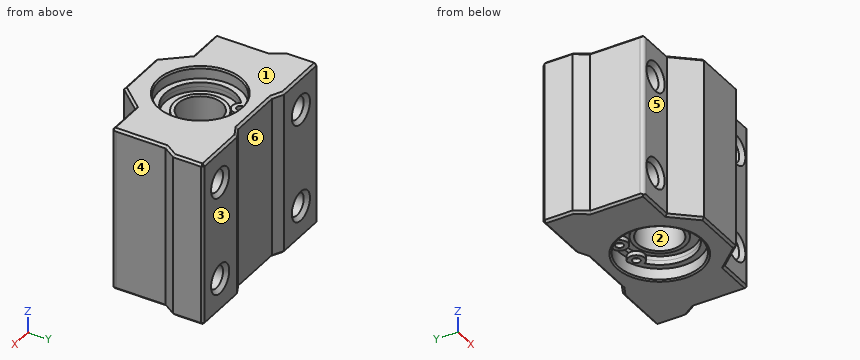
```python
from build123d import *

# Parameters (mm, degrees)
SKETCH1_R             = 7.5
BOSS_EXTRUDE1_DEPTH   = 15
SKETCH3_R             = 0.7
BOSS_EXTRUDE2_DEPTH   = 0.8
CHAFL_N0_SIZE         = 0.2
CHAFL_N0_SIZE2        = 0.346410162
CHAFL_N0_PART_2_SIZE  = 0.2
CHAFL_N0_PART_2_SIZE2 = 0.346410162
CROQUIS1_R            = 2
CORTAR_EXTRUIR1_DEPTH = 20
CHAFL_N1_SIZE         = 0.7
CHAFL_N2_SIZE         = 0.4
REDONDEO1_R           = 0.7


with BuildPart() as part:
    # Sketch1 → Boss-Extrude1 (new body, symmetric)
    with BuildSketch(Plane.XY):
        Polygon((-5, -1), (5, -1), (7, 0), (17, 0), (17, -5.5), (15.5, -7.8), (15.5, -17.6), (8.6, -17.6), (4.75, -22), (-4.75, -22), (-8.6, -17.6), (-15.5, -17.6), (-15.5, -7.8), (-17, -5.5), (-17, 0), (-7, 0), align=None)
        with Locations((0, -11)):
            Circle(SKETCH1_R, mode=Mode.SUBTRACT)
    extrude(amount=BOSS_EXTRUDE1_DEPTH, both=True)

    # Sketch2 → Revolve1 (revolve)
    with BuildSketch(Plane(origin=(0, 0, 0), x_dir=(0, 0, -1), z_dir=(1, 0, 0))):
        Polygon((-12, -3.5), (12, -3.5), (12, -4.6), (11.2, -4.6), (11.2, -6.3), (11.8, -6.3), (11.8, -7), (-11.8, -7), (-11.8, -6.3), (-11.2, -6.3), (-11.2, -4.6), (-12, -4.6), align=None)
    revolve(axis=Axis((0, -11, 30.2753079), (0, 0, -1)))

    # Sketch3 → Boss-Extrude2 (add)
    with BuildSketch(Plane.XY.offset(12)):
        with BuildLine():
            ThreePointArc((2, -3.771583853), (1.369159148, -6.17129169), (3.832579259, -5.874442838))
            ThreePointArc((3.832579259, -5.874442838), (0, -17.4), (-3.832579259, -5.874442838))
            ThreePointArc((-3.832579259, -5.874442838), (-1.369159148, -6.17129169), (-2, -3.771583853))
            ThreePointArc((-2, -3.771583853), (0, -18.5), (2, -3.771583853))
        make_face()
        with Locations((2.5, -5.185797415)):
            Circle(SKETCH3_R, mode=Mode.SUBTRACT)
        with Locations((-2.5, -5.185797415)):
            Circle(SKETCH3_R, mode=Mode.SUBTRACT)
    boss_extrude2 = extrude(amount=BOSS_EXTRUDE2_DEPTH)

    # simetria: Boss-Extrude2 across plane
    add(boss_extrude2.mirror(Plane.XY))

    # Chaflàn0
    chafl_n0_edges = [part.edges().sort_by_distance(p)[0] for p in [
        (-7.5, -11, -15),
    ]]
    chafl_n0_side = [part.faces().sort_by_distance(p)[0] for p in [
        (-7.5, -11, -13.5),
    ]]
    chamfer(chafl_n0_edges, length=CHAFL_N0_SIZE, length2=CHAFL_N0_SIZE2, reference=chafl_n0_side[0])

    # Chaflàn0 part 2
    chafl_n0_part_2_edges = [part.edges().sort_by_distance(p)[0] for p in [
        (-7.5, -11, 15),
    ]]
    chafl_n0_part_2_side = [part.faces().sort_by_distance(p)[0] for p in [
        (0, -1.404969135, 15),
    ]]
    chamfer(chafl_n0_part_2_edges, length=CHAFL_N0_PART_2_SIZE, length2=CHAFL_N0_PART_2_SIZE2, reference=chafl_n0_part_2_side[0])

    # Croquis1 → Cortar-Extruir1 (cut)
    with BuildSketch(Plane(origin=(0, 0, 0), x_dir=(1, 0, 0), z_dir=(0, 1, 0))):
        with Locations((-12, 9)):
            Circle(CROQUIS1_R)
        with Locations((12, 9)):
            Circle(CROQUIS1_R)
        with Locations((-12, -9)):
            Circle(CROQUIS1_R)
        with Locations((12, -9)):
            Circle(CROQUIS1_R)
    extrude(amount=-CORTAR_EXTRUIR1_DEPTH, mode=Mode.SUBTRACT)

    # Chaflán1
    chafl_n1_edges = [part.edges().sort_by_distance(p)[0] for p in [
        (-14, -17.6, -9),
        (-14, 0, -9),
        (10, -17.6, -9),
        (10, 0, -9),
        (-14, -17.6, 9),
        (-14, 0, 9),
        (10, -17.6, 9),
        (10, 0, 9),
    ]]
    chamfer(chafl_n1_edges, length=CHAFL_N1_SIZE)

    # Chaflán2
    chafl_n2_edges = [part.edges().sort_by_distance(p)[0] for p in [
        (-6, -0.5, 15),
        (-12, 0, 15),
        (12, 0, -15),
        (17, -2.75, -15),
        (16.25, -6.65, -15),
        (15.5, -12.7, -15),
        (12.05, -17.6, -15),
        (-17, -2.75, 15),
        (6.675, -19.8, -15),
        (0, -22, -15),
        (-6.675, -19.8, -15),
        (-12.05, -17.6, -15),
        (-15.5, -12.7, -15),
        (-16.25, -6.65, -15),
        (-17, -2.75, -15),
        (-12, 0, -15),
        (-16.25, -6.65, 15),
        (-6, -0.5, -15),
        (0, -1, -15),
        (6, -0.5, -15),
        (-15.5, -12.7, 15),
        (-12.05, -17.6, 15),
        (17, 0, 0),
        (-17, 0, 0),
        (-6.675, -19.8, 15),
        (0, -22, 15),
        (6.675, -19.8, 15),
        (12.05, -17.6, 15),
        (6, -0.5, 15),
        (15.5, -12.7, 15),
        (16.25, -6.65, 15),
        (17, -2.75, 15),
        (12, 0, 15),
        (0, -1, 15),
    ]]
    chamfer(chafl_n2_edges, length=CHAFL_N2_SIZE)

    # Redondeo1
    redondeo1_edges = [part.edges().sort_by_distance(p)[0] for p in [
        (15.5, -17.6, 0),
        (-15.5, -17.6, 0),
    ]]
    fillet(redondeo1_edges, radius=REDONDEO1_R)


solid = part.part
```
For this review, take the finished solid that the model builds, in its own axes (mm). Face numbers are marked on the shaded views. A direction names the side the tool comes from. Round coordinates to 2 decimals unless told otherwise and drop trailing zeros. Order: outer loops, then holes, each group sorted by start corner. A loop starts at its lowest first (then second) coordinate and runs counter-clockwise, first axis right, second up.
Q1. Wall thickness on line 1 (X direction, y = -11, z = -13.4); line 2 (X direction, y = -10, z = -8); line 3 (Z direction, x = 11.5, y = -14.75): over which ranges is each line inside the solid? List them lowest first.
Findings below:
line 1: x = -15.5 to -7.5, 7.5 to 15.5
line 2: x = -15.5 to -13.73, -10.27 to -3.87, 3.87 to 10.27, 13.73 to 15.5
line 3: z = -15 to -10.94, -7.06 to 7.06, 10.94 to 15
Q2. We need section B-B, the plane z = 5. Give the boundary of the cut face in (x, y).
Findings below:
outline: (-17, -5.5) - (-15.5, -7.8) - (-15.5, -16.9) arc R0.7 ccw to (-14.8, -17.6) - (-8.6, -17.6) - (-4.75, -22) - (4.75, -22) - (8.6, -17.6) - (14.8, -17.6) arc R0.7 ccw to (15.5, -16.9) - (15.5, -7.8) - (17, -5.5) - (17, -0.4) - (16.6, 0) - (7, 0) - (5, -1) - (-5, -1) - (-7, 0) - (-16.6, 0) - (-17, -0.4) - close; hole circle Ø8 at (0, -11)
Q3. Mouldability with a two-part tool opening along Y and no side actions: class the marked faces 1, 2 and 3 as pulls with the +Y half, pulls with the -Y half, needs draft (parallel to the pull), parting line crosses it, or undercut.
Findings below:
face 1: needs draft
face 2: undercut
face 3: pulls with the +Y half
Q4. Machinability: for the marked faces 4, 5 and 6, which of the approach directions +Z, -Z, +X, -X, +Y, -Y give a long, thin tool a straight path to every point of the face, cutting with its end or side? Answer none if there is none.
Findings below:
face 4: +Z, -Z, +X, -Y
face 5: +Z, -Z, -X, -Y
face 6: +Z, -Z, +Y
Q5. Insertion check: P1, Ø4.5, axis at x = -12, z = -9, coming from the -Y side; P2, Ø12, axis at y = -18, z = -11.5, coming from the +X side; P3, Ø10, axis at y = -11, z = -8.5, coming from the +X side. Each pin has a flat end and moves straight along its axis. Give the tip position at first contact, or say it passes through.
Findings below:
P1: stops at y = -17.15
P2: stops at x = 15.5
P3: stops at x = 16.67
Q6. We need section A-A, the plane x = -12. Give the boundary of the cut face in (y, z), plus the area to 3 significant figures.
Findings below:
outline: (-17.6, -14.6) - (-17.2, -15) - (-0.4, -15) - (0, -14.6) - (0, -11.7) - (-0.7, -11) - (-16.9, -11) - (-17.6, -11.7) - close; (-17.6, -6.3) - (-16.9, -7) - (-0.7, -7) - (0, -6.3) - (0, 6.3) - (-0.7, 7) - (-16.9, 7) - (-17.6, 6.3) - close; (-17.6, 11.7) - (-16.9, 11) - (-0.7, 11) - (0, 11.7) - (0, 14.6) - (-0.4, 15) - (-17.2, 15) - (-17.6, 14.6) - close
area: 385 mm2
Q7. We need section C-C, the plane y = -11. State how many separate pieces and enclosed holes the cut face has, plus the area to 3 significant figures.
Findings below:
separate pieces: 2
enclosed holes: 4
area: 595 mm2
